```python
from build123d import *

# Parameters (mm, degrees)
SKETCH1_W              = 150
SKETCH1_H              = 50
BODY_DEPTH             = 4
EDGE_FILLETS_R         = 5
GX16_HOLE_D            = 16.5
GX16_PATTERN_COUNT     = 4
GX16_PATTERN_PITCH     = 35
DESIGN_CUTOUT_SKETCH_W = 0.641025641
DESIGN_CUTOUT_SKETCH_H = 5
DESIGN_CUTOUT_DEPTH    = 0.5


# Read off the part's stored shape, not the designer's step: mounting_holes
with BuildPart() as part:
    # Sketch1 → body (new body)
    with BuildSketch(Plane(origin=(0, 0, 0), x_dir=(1, 0, 0), z_dir=(0, 1, 0))):
        Rectangle(SKETCH1_W, SKETCH1_H)
    extrude(amount=BODY_DEPTH)

    # mounting_holes outline → mounting_holes (revolve, cut)
    with BuildSketch(Plane(origin=(70, 0, 20), x_dir=(1, 0, 0), z_dir=(0, 0, 1))):
        Polygon((0, 0), (1.7, 0), (1.7, 2), (3.25, 2), (3.25, 3.975), (3.275, 4), (0, 4), align=None)
    revolve(axis=Axis((70, 0, 20), (0, 1, 0)), mode=Mode.SUBTRACT)

    # mounting_holes 2 outline → mounting_holes 2 (revolve, cut)
    with BuildSketch(Plane(origin=(-70, 0, -20), x_dir=(1, 0, 0), z_dir=(0, 0, 1))):
        Polygon((0, 4), (0, 0), (1.7, 0), (1.7, 2), (3.25, 2), (3.25, 3.975), (3.275, 4), align=None)
    revolve(axis=Axis((-70, 0, -20), (0, 1, 0)), mode=Mode.SUBTRACT)

    # mounting_holes 3 outline → mounting_holes 3 (revolve, cut)
    with BuildSketch(Plane(origin=(70, 0, -20), x_dir=(1, 0, 0), z_dir=(0, 0, 1))):
        Polygon((0, 4), (0, 0), (1.7, 0), (1.7, 2), (3.25, 2), (3.25, 3.975), (3.275, 4), align=None)
    revolve(axis=Axis((70, 0, -20), (0, 1, 0)), mode=Mode.SUBTRACT)

    # mounting_holes 4 outline → mounting_holes 4 (revolve, cut)
    with BuildSketch(Plane(origin=(-70, 0, 20), x_dir=(1, 0, 0), z_dir=(0, 0, 1))):
        Polygon((0, 4), (0, 0), (1.7, 0), (1.7, 2), (3.25, 2), (3.25, 3.975), (3.275, 4), align=None)
    revolve(axis=Axis((-70, 0, 20), (0, 1, 0)), mode=Mode.SUBTRACT)

    # edge_fillets
    edge_fillets_edges = [part.edges().sort_by_distance(p)[0] for p in [
        (75, 2, 25),
        (-75, 2, 25),
        (-75, 2, -25),
        (75, 2, -25),
    ]]
    fillet(edge_fillets_edges, radius=EDGE_FILLETS_R)

    # gx16_hole (through all)
    with Locations(Plane(origin=(0, 4, 0), x_dir=(1, 0, 0), z_dir=(0, 1, 0))):
        with Locations((-52.5, 0)):
            gx16_hole = Hole(GX16_HOLE_D / 2)

    # gx16_pattern: gx16_hole ×4
    with Locations(*[(i * GX16_PATTERN_PITCH, 0, 0) for i in range(1, GX16_PATTERN_COUNT)]):
        add(gx16_hole, mode=Mode.SUBTRACT)

    # design_cutout_sketch → design_cutout (cut)
    with BuildSketch(Plane(origin=(0, 4, 0), x_dir=(1, 0, 0), z_dir=(0, 1, 0))):
        with BuildLine():
            Line((-34.5, 15), (-34.5, -15))
            ThreePointArc((-34.5, -15), (-35, -15.5), (-35.5, -15))
            Line((-35.5, -15), (-35.5, 15))
            ThreePointArc((-35.5, 15), (-35, 15.5), (-34.5, 15))
        make_face()
        with BuildLine():
            Line((0.5, 15), (0.5, -15))
            ThreePointArc((0.5, -15), (0, -15.5), (-0.5, -15))
            Line((-0.5, -15), (-0.5, 15))
            ThreePointArc((-0.5, 15), (0, 15.5), (0.5, 15))
        make_face()
        with BuildLine():
            Line((35.5, 15), (35.5, -15))
            ThreePointArc((35.5, -15), (35, -15.5), (34.5, -15))
            Line((34.5, -15), (34.5, 15))
            ThreePointArc((34.5, 15), (35, 15.5), (35.5, 15))
        make_face()
        with Locations((-52.403846154, 17.5)):
            Rectangle(DESIGN_CUTOUT_SKETCH_W, DESIGN_CUTOUT_SKETCH_H)
        with Locations((-18.46923077, 17.5)):
            Rectangle(DESIGN_CUTOUT_SKETCH_W, DESIGN_CUTOUT_SKETCH_H)
        with Locations((-16.674358975, 17.5)):
            Rectangle(DESIGN_CUTOUT_SKETCH_W, DESIGN_CUTOUT_SKETCH_H)
        with Locations((15.711538462, 17.5)):
            Rectangle(DESIGN_CUTOUT_SKETCH_W, DESIGN_CUTOUT_SKETCH_H)
        with Locations((17.506410257, 17.5)):
            Rectangle(DESIGN_CUTOUT_SKETCH_W, DESIGN_CUTOUT_SKETCH_H)
        with Locations((19.301282052, 17.5)):
            Rectangle(DESIGN_CUTOUT_SKETCH_W, DESIGN_CUTOUT_SKETCH_H)
        with Locations((50.711538462, 17.5)):
            Rectangle(DESIGN_CUTOUT_SKETCH_W, DESIGN_CUTOUT_SKETCH_H)
        Polygon((51.737179487, 20), (52.382211538, 20), (53.976762821, 16.166866987), (55.571314103, 20), (56.224358974, 20), (54.079927885, 15), (53.874599359, 15), align=None)
    extrude(amount=-DESIGN_CUTOUT_DEPTH, mode=Mode.SUBTRACT)


solid = part.part
```
Geometry: final body of the model. Coordinates: model frame, mm. A direction names the side the tool comes from. Round coordinates to 2 decimals unless told otherwise and drop trailing zeros. Order: outer loops, then holes, each group sorted by start corner. A loop starts at its lowest first (then second) coordinate and runs counter-clockwise, first axis right, second up. Notation, with made-up numbers: M 89.5,58 L 145.5,58 A27 cw 145.5,90 Z; hole C 35.25,-6 d4. An arc over 180 degrees is marked long. Use one line per item in the form item = value. Start each with the question number.
Q1. Access query for faces 1 (the face through (73, 2, 24)), 2 (the face through (-71.4, 2, -18.6)). Directions: +Z, -Z, +X, -X, +Y, -Y. A direction counts if a zero-diameter tool reaches every point of the face in a straight line with its end or side. Return the directions, or none.
Q2. Material intervals for line 1 (Z direction, x = -70, y = 1.15); line 2 (Z direction, x = 70, y = 3.35); line 3 (X direction, y = 1, z = -0.5), sorted ascending. Write a range as [from, to].
Q3. Cut plane A-A (z = 0). Count the separate pieces of the cut face and the enclosed holes in it, and give its area (4 significant figures).
Q4. Cut plane C-C (x = 11). Return loops of the section in (y, z).
Q5. Mould query, pull axis X, two halves, no side actions, for faces 3 (the face through (-74, 2, -23)), 4 (the face through (-1, 0, 0)), 5 (the face through (-9.258, 1.972, -0.363)). Classes: +X half, -X half, draft (parallel to the pull), parting line (faces both ways), or undercut.
Q6. Cut plane B-B (x = -47). Return loops of the section in (y, z).
Geometry results:
q1.face_1 = +Z, +X, +Y, -Y
q1.face_2 = +Y
q2.line_1 = [-25, -21.7], [-18.3, 18.3], [21.7, 25]
q2.line_2 = [-25, -23.25], [-16.75, 16.75], [23.25, 25]
q2.line_3 = [-75, -60.73], [-44.27, -25.73], [-9.27, 9.27], [25.73, 44.27], [60.73, 75]
q3.separate_pieces = 5
q3.enclosed_holes = 0
q3.area = 334.5 mm^2
q4.outline = M 0,-25 L 4,-25 L 4,-5.08 L 0,-5.08 Z; M 0,5.08 L 4,5.08 L 4,25 L 0,25 Z
q5.face_3 = -X half
q5.face_4 = draft
q5.face_5 = undercut
q6.outline = M 0,-25 L 4,-25 L 4,-6.15 L 0,-6.15 Z; M 0,6.15 L 4,6.15 L 4,25 L 0,25 Z
